Could you check a few things on this model? Use its own coordinates, in mm. Round coordinates to 2 decimals unless told otherwise and drop trailing zeros. Loops run counter-clockwise (first coordinate to the right, second up) from the corner with the lowest first, then second, coordinate; pieces in that order, holes last.
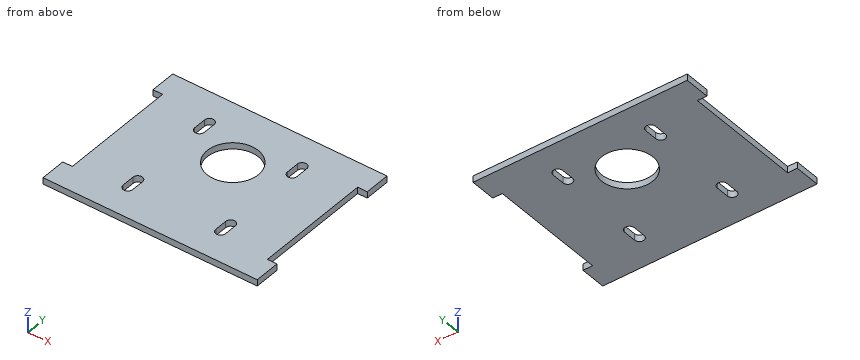
from build123d import *

# Parameters (mm, degrees)
SKETCH2_W          = 212.725
SKETCH2_H          = 166.909166922
EXTRUDE1_DEPTH     = 6.35
CUT_EXTRUDE1_REACH = 152.519
SKETCH3_R          = 25.4
CUT_EXTRUDE2_REACH = 152.519
SKETCH4_W          = 9.525
SKETCH4_H          = 116.109166922


with BuildPart() as part:
    # Sketch2 → Extrude1 (new body)
    with BuildSketch(Plane.XY):
        with Locations((0, -22.86)):
            Rectangle(SKETCH2_W, SKETCH2_H)
    extrude(amount=EXTRUDE1_DEPTH)

    # Sketch3 → Cut-Extrude1 (cut, up to next)
    with BuildSketch(Plane.XY.offset(6.35), mode=Mode.PRIVATE) as cut_extrude1_sk1:
        Circle(SKETCH3_R)
    cut_extrude1_tool1 = extrude(cut_extrude1_sk1.sketch, amount=-CUT_EXTRUDE1_REACH, mode=Mode.PRIVATE) & part.part
    # Sketch3 → Cut-Extrude1 (cut, up to next)
    with BuildSketch(Plane.XY.offset(6.35), mode=Mode.PRIVATE) as cut_extrude1_sk2:
        with BuildLine():
            Line((50.8, -75.2475), (50.8, -62.5475))
            ThreePointArc((50.8, -62.5475), (46.0375, -57.785), (41.275, -62.5475))
            Line((41.275, -62.5475), (41.275, -75.2475))
            ThreePointArc((41.275, -75.2475), (46.0375, -80.01), (50.8, -75.2475))
        make_face()
    cut_extrude1_tool2 = extrude(cut_extrude1_sk2.sketch, amount=-CUT_EXTRUDE1_REACH, mode=Mode.PRIVATE) & part.part
    # Sketch3 → Cut-Extrude1 (cut, up to next)
    with BuildSketch(Plane.XY.offset(6.35), mode=Mode.PRIVATE) as cut_extrude1_sk3:
        with BuildLine():
            Line((50.8, 16.8275), (50.8, 29.5275))
            ThreePointArc((50.8, 29.5275), (46.0375, 34.29), (41.275, 29.5275))
            Line((41.275, 29.5275), (41.275, 16.8275))
            ThreePointArc((41.275, 16.8275), (46.0375, 12.065), (50.8, 16.8275))
        make_face()
    cut_extrude1_tool3 = extrude(cut_extrude1_sk3.sketch, amount=-CUT_EXTRUDE1_REACH, mode=Mode.PRIVATE) & part.part
    # Sketch3 → Cut-Extrude1 (cut, up to next)
    with BuildSketch(Plane.XY.offset(6.35), mode=Mode.PRIVATE) as cut_extrude1_sk4:
        with BuildLine():
            Line((-41.275, 16.8275), (-41.275, 29.5275))
            ThreePointArc((-41.275, 29.5275), (-46.0375, 34.29), (-50.8, 29.5275))
            Line((-50.8, 29.5275), (-50.8, 16.8275))
            ThreePointArc((-50.8, 16.8275), (-46.0375, 12.065), (-41.275, 16.8275))
        make_face()
    cut_extrude1_tool4 = extrude(cut_extrude1_sk4.sketch, amount=-CUT_EXTRUDE1_REACH, mode=Mode.PRIVATE) & part.part
    # Sketch3 → Cut-Extrude1 (cut, up to next)
    with BuildSketch(Plane.XY.offset(6.35), mode=Mode.PRIVATE) as cut_extrude1_sk5:
        with BuildLine():
            Line((-41.275, -75.2475), (-41.275, -62.5475))
            ThreePointArc((-41.275, -62.5475), (-46.0375, -57.785), (-50.8, -62.5475))
            Line((-50.8, -62.5475), (-50.8, -75.2475))
            ThreePointArc((-50.8, -75.2475), (-46.0375, -80.01), (-41.275, -75.2475))
        make_face()
    cut_extrude1_tool5 = extrude(cut_extrude1_sk5.sketch, amount=-CUT_EXTRUDE1_REACH, mode=Mode.PRIVATE) & part.part
    add(cut_extrude1_tool1.solids().sort_by_distance((0, 0, 6.35))[0], mode=Mode.SUBTRACT)
    add(cut_extrude1_tool2.solids().sort_by_distance((46.0375, -68.8975, 6.35))[0], mode=Mode.SUBTRACT)
    add(cut_extrude1_tool3.solids().sort_by_distance((46.0375, 23.1775, 6.35))[0], mode=Mode.SUBTRACT)
    add(cut_extrude1_tool4.solids().sort_by_distance((-46.0375, 23.1775, 6.35))[0], mode=Mode.SUBTRACT)
    add(cut_extrude1_tool5.solids().sort_by_distance((-46.0375, -68.8975, 6.35))[0], mode=Mode.SUBTRACT)

    # Sketch4 → Cut-Extrude2 (cut, up to next)
    with BuildSketch(Plane.XY.offset(6.35), mode=Mode.PRIVATE) as cut_extrude2_sk1:
        with Locations((-101.6, -22.86)):
            Rectangle(SKETCH4_W, SKETCH4_H)
    cut_extrude2_tool1 = extrude(cut_extrude2_sk1.sketch, amount=-CUT_EXTRUDE2_REACH, mode=Mode.PRIVATE) & part.part
    # Sketch4 → Cut-Extrude2 (cut, up to next)
    with BuildSketch(Plane.XY.offset(6.35), mode=Mode.PRIVATE) as cut_extrude2_sk2:
        with Locations((101.6, -22.86)):
            Rectangle(SKETCH4_W, SKETCH4_H)
    cut_extrude2_tool2 = extrude(cut_extrude2_sk2.sketch, amount=-CUT_EXTRUDE2_REACH, mode=Mode.PRIVATE) & part.part
    add(cut_extrude2_tool1.solids().sort_by_distance((-101.6, -22.86, 6.35))[0], mode=Mode.SUBTRACT)
    add(cut_extrude2_tool2.solids().sort_by_distance((101.6, -22.86, 6.35))[0], mode=Mode.SUBTRACT)


solid = part.part
Item 1: Will these pins go through, and if not, where does the flat tip stop? pin 1 (1.9 mm diameter, centred on y = -38, z = 4.5, fed in from -X); pin 2 (2 mm diameter, centred on y = -56.5, z = 5, fed in from +X).
Results list:
pin 1: stops at x = -96.84
pin 2: stops at x = 96.84
Item 2: If we section it at B-B, the plane y = 0: Please give me the cut outline in (x, z), then the cut area to 3 significant figures.
Results list:
outline: (-96.84, 0) - (-25.4, 0) - (-25.4, 6.35) - (-96.84, 6.35) - close; (25.4, 0) - (96.84, 0) - (96.84, 6.35) - (25.4, 6.35) - close
area: 907 mm2
Item 3: If we section it at D-D, the plane z = 2.25: Count the separate pieces of the cut face and the enclosed holes in it, then the cut area to 3 significant figures.
Results list:
separate pieces: 1
enclosed holes: 5
area: 30,500 mm2
Item 4: If I drill on line 1 along X through (y, z) = (-64, 4.5) (1 decimal); line 2 along X through (y, z) = (-61, 3.25); line 3 along Y through (x, z) = (-47, 1), over which ranges is the centre line in solid material (lowest first)?
Results list:
line 1: x = -96.8 to -50.8, -41.3 to 41.3, 50.8 to 96.8
line 2: x = -96.84 to -50.54, -41.53 to 41.53, 50.54 to 96.84
line 3: y = -106.31 to -79.91, -57.88 to 12.16, 34.19 to 60.59
Item 5: If we section it at C-C, the plane x = -15.5: Please give me the cut outline in (y, z), then the cut area to 3 significant figures.
Results list:
outline: (-106.31, 0) - (-20.12, 0) - (-20.12, 6.35) - (-106.31, 6.35) - close; (20.12, 0) - (60.59, 0) - (60.59, 6.35) - (20.12, 6.35) - close
area: 804 mm2
Item 6: If we section it at A-A, the plane x = 48: Please give me the cut outline in (y, z).
Results list:
outline: (-106.31, 0) - (-79.59, 0) - (-79.59, 6.35) - (-106.31, 6.35) - close; (-58.21, 0) - (12.49, 0) - (12.49, 6.35) - (-58.21, 6.35) - close; (33.87, 0) - (60.59, 0) - (60.59, 6.35) - (33.87, 6.35) - close
